from build123d import *

# Parameters (mm, degrees)
SKETCH1_W          = 76.454
SKETCH1_H          = 56.007
EXTRUDE1_DEPTH     = 1.5875
SKETCH2_R          = 0.8128
EXTRUDE2_DEPTH     = 95.786699073
SKETCH4_R          = 0.8128
EXTRUDE3_DEPTH     = 9.525
SKETCH5_W          = 3.048
SKETCH5_H          = 19.05
EXTRUDE4_DEPTH     = 95.786699073
SKETCH6_R          = 0.8128
CUT_EXTRUDE1_DEPTH = 1.5875


with BuildPart() as part:
    # Sketch1 → Extrude1 (new body)
    with BuildSketch(Plane.XY):
        with Locations((-38.227, 28.0035)):
            Rectangle(SKETCH1_W, SKETCH1_H)
    extrude(amount=-EXTRUDE1_DEPTH)

    # Sketch2 → Extrude2 (cut, through all)
    with BuildSketch(Plane.XY):
        with Locations((-38.227, 54.42458)):
            Circle(SKETCH2_R)
        with Locations((-30.607, 54.42458)):
            Circle(SKETCH2_R)
        with Locations((-22.987, 54.42458)):
            Circle(SKETCH2_R)
        with Locations((-15.367, 54.42458)):
            Circle(SKETCH2_R)
        with Locations((-45.847, 54.42458)):
            Circle(SKETCH2_R)
        with Locations((-53.467, 54.42458)):
            Circle(SKETCH2_R)
        with Locations((-61.087, 54.42458)):
            Circle(SKETCH2_R)
    extrude(amount=-EXTRUDE2_DEPTH, mode=Mode.SUBTRACT)

    # Sketch4 → Extrude3 (cut)
    with BuildSketch(Plane.XY):
        with Locations((-75.16495, 26.416)):
            Circle(SKETCH4_R)
        with Locations((-75.16495, 18.796)):
            Circle(SKETCH4_R)
        with Locations((-1.28905, 26.416)):
            Circle(SKETCH4_R)
        with Locations((-1.28905, 18.796)):
            Circle(SKETCH4_R)
    extrude(amount=-EXTRUDE3_DEPTH, mode=Mode.SUBTRACT)

    # Sketch5 → Extrude4 (cut, through all)
    with BuildSketch(Plane.XY):
        with Locations((-74.93, 46.482)):
            Rectangle(SKETCH5_W, SKETCH5_H)
        with Locations((-1.524, 46.482)):
            Rectangle(SKETCH5_W, SKETCH5_H)
    extrude(amount=-EXTRUDE4_DEPTH, mode=Mode.SUBTRACT)

    # Sketch6 → Cut-Extrude1 (cut)
    with BuildSketch(Plane.XY):
        with Locations((-12.827, 2.20853)):
            Circle(SKETCH6_R)
        with Locations((-63.766480146, 2.20853)):
            Circle(SKETCH6_R)
    extrude(amount=-CUT_EXTRUDE1_DEPTH, mode=Mode.SUBTRACT)


solid = part.part
The listing builds one solid part. Answer for the finished solid, in the listing's coordinates (mm). A direction names the side the tool comes from. Give positions to 0.01 mm unless a question says otherwise; leave off trailing zeros. Loops run counter-clockwise (first coordinate to the right, second up) from the corner with the lowest first, then second, coordinate; pieces in that order, holes last.
Item 1: Find the intervals of material crossed by line 1 along X through (y, z) = (38.5, -0.45); line 2 along Y through (x, z) = (-23, -0.25), in increasing order.
Derived:
line 1: x = -73.41 to -3.05
line 2: y = 0 to 53.61, 55.24 to 56.01
Item 2: A tool of negligible diameter and unlimited length cuts with its end or side. For faces 1 (the flat face through (-73.406, 46, -1)), 2 (the flat face through (-3.048, 46, -1)), 3 (the cylindrical face through (-54.11, 53.93, -0.78)), from which of +Z, -Z, +X, -X, +Y, -Y can it reach the whole face along a straight path? Write none if from no direction.
Derived:
face 1: +Z, -Z, -X, +Y
face 2: +Z, -Z, +X, +Y
face 3: +Z, -Z
Item 3: A cutting plane is placed at B-B (y = 41). Give the vertices of the cut face in (x, z), then the cut area to 3 significant figures.
Derived:
outline: (-73.41, -1.59) - (-3.05, -1.59) - (-3.05, 0) - (-73.41, 0) - close
area: 112 mm2
Item 4: Each of these flat-tipped pins is pushed along its axis until it touches: pin 1 Ø0.5 at (x, z) = (-75.5, -1) entering from +Y; pin 2 Ø1.5 at (x, y) = (-75.16, 26.42) entering from +Z; pin 3 Ø0.8 at (y, z) = (46.5, -0.5) entering from +X. Where does it stop, or does it pass through?
Derived:
pin 1: stops at y = 36.96
pin 2: passes through
pin 3: stops at x = -3.05
Item 5: Determine the mould class of faces 4 (the flat face through (-39, 28, 0)), 5 (the flat face through (-2, 36.957, -1)), 6 (the cylindrical face through (-12.076, 1.897, -0.783)) for opening direction Y: +Y half, -Y half, draft (parallel to the pull), parting line (faces both ways), or undercut.
Derived:
face 4: draft
face 5: +Y half
face 6: undercut
Item 6: A cutting plane is placed at A-A (z = -0.45). Give the number of separate pieces and of enclosed holes in the cut face, then the cut area to 3 significant figures.
Derived:
separate pieces: 1
enclosed holes: 13
area: 4,140 mm2
